Verification items for the finished model (mm, model axes). A direction names the side the tool comes from. Round coordinates to 2 decimals unless told otherwise and drop trailing zeros. Order: outer loops, then holes, each group sorted by start corner. A loop starts at its lowest first (then second) coordinate and runs counter-clockwise, first axis right, second up.
```python
from build123d import *

# Parameters (mm, degrees)
BOSS_EXTRUDE1_DEPTH = 500
SKETCH5_R           = 1.5
CUT_EXTRUDE1_DEPTH  = 5
SKETCH6_W           = 76.2
SKETCH6_H           = 76.2
BOSS_EXTRUDE2_DEPTH = 9.144
SKETCH7_R           = 1.65
CUT_EXTRUDE2_DEPTH  = 9.144
FILLET1_R           = 5


with BuildPart() as part:
    # Sketch3 → Boss-Extrude1 (new body)
    with BuildSketch(Plane(origin=(0, 0, 0), x_dir=(1, 0, 0), z_dir=(0, 1, 0))):
        with BuildLine():
            Line((-10, -16.214268408), (10, -16.214268408))
            ThreePointArc((10, -16.214268408), (0, 19.05), (-10, -16.214268408))
        make_face()
    extrude(amount=BOSS_EXTRUDE1_DEPTH)

    # Sketch5 → Cut-Extrude1 (cut)
    with BuildSketch(Plane.XY.offset(16.214268408)):
        with Locations((0, 321.4)):
            Circle(SKETCH5_R)
    extrude(amount=-CUT_EXTRUDE1_DEPTH, mode=Mode.SUBTRACT)

    # Sketch6 → Boss-Extrude2 (add)
    with BuildSketch(Plane.XZ):
        Rectangle(SKETCH6_W, SKETCH6_H)
    extrude(amount=BOSS_EXTRUDE2_DEPTH)

    # Sketch7 → Cut-Extrude2 (cut)
    with BuildSketch(Plane.XZ.offset(9.144)):
        with Locations((-25, 25)):
            Circle(SKETCH7_R)
        with Locations((25, 25)):
            Circle(SKETCH7_R)
        with Locations((25, -25)):
            Circle(SKETCH7_R)
        with Locations((-25, -25)):
            Circle(SKETCH7_R)
    extrude(amount=-CUT_EXTRUDE2_DEPTH, mode=Mode.SUBTRACT)

    # Fillet1
    fillet1_edges = [part.edges().sort_by_distance(p)[0] for p in [
        (38.1, -4.572, -38.1),
        (38.1, -4.572, 38.1),
        (-38.1, -4.572, 38.1),
        (-38.1, -4.572, -38.1),
    ]]
    fillet(fillet1_edges, radius=FILLET1_R)


solid = part.part
```
1) Sectioned sample at B-B on y = 102. Record the cut outline in (x, z).
2) Tool access check on faces 1 (the flat face through (0, 500, -2)), 2 (the flat face through (0, 246, 16.214)), 3 (the flat face through (-1, 0, 17)). Record the directions out of +Z, -Z, +X, -X, +Y, -Y that give a thin tool (end or side, any length) a straight path to the whole face; none if there is none.
3) Sectioned sample at A-A on z = 0. Record the cut outline in (x, y), then the cut area to 3 significant figures.
4) Scan lines: probe 1 along Z at (x, y) = (25, -5); probe 2 along Y at (x, z) = (28, -35); probe 3 along X at (y, z) = (321.4, 13.2). Record each from-to range of solid material in increasing order.
5) Go/stop test with flat-tipped pins: pin 1 Ø10 at (y, z) = (50.5, -10.5) entering from -X; pin 2 Ø4 at (x, y) = (16, 98.5) entering from -Z; pin 3 Ø4.5 at (x, z) = (25, 25) entering from -Y; pin 4 Ø0.9 at (x, y) = (-0.5, 321) entering from +Z. Record where each tip stops, or that it passes through.
Returned:
1. outline: (-10, 16.21) arc R19.05 ccw (long way) to (10, 16.21) - close
2. face 1: +Z, -Z, +X, -X, +Y
2. face 2: +Z, +X, -X, +Y
2. face 3: +Y
3. outline: (-38.1, -9.14) - (38.1, -9.14) - (38.1, 0) - (19.05, 0) - (19.05, 500) - (-19.05, 500) - (-19.05, 0) - (-38.1, 0) - close
3. area: 19,700 mm2
4. probe 1: z = -38.1 to -26.65, -23.35 to 23.35, 26.65 to 38.1
4. probe 2: y = -9.14 to 0
4. probe 3: x = -13.74 to -1.5, 1.5 to 13.74
5. pin 1: stops at x = -18.24
5. pin 2: stops at z = -12.92
5. pin 3: stops at y = -9.14
5. pin 4: stops at z = 11.21
